from build123d import *

# Parameters (mm, degrees)
SKETCH1_R           = 3.1
BOSS_EXTRUDE1_DEPTH = 6


with BuildPart() as part:
    # Sketch1 → Boss-Extrude1 (new body)
    with BuildSketch(Plane(origin=(0, 0, 0), x_dir=(1, 0, 0), z_dir=(0, 1, 0))):
        with BuildLine():
            ThreePointArc((-31.599916308, 0.035666759), (-29.38660688, -5.361386604), (-24, -7.6))
            add(Edge.make_bspline(
                [(-24, -7.6), (-14.668264125, -7.61499575), (0.011178466, 17.82220608), (14.645907193, -7.566074292), (24, -7.6)],
                knots=[0, 0, 0, 0, 0.5, 1, 1, 1, 1], degree=3))
            ThreePointArc((24, -7.6), (29.374011537, -5.374011537), (31.6, 0))
            add(Edge.make_bspline(
                [(-31.599916308, 0.035666759), (-31.577855131, 6.453958953), (-15.873953038, 23.775800665), (16.019610489, 23.704017602), (31.552058953, 7.12035463), (31.6, 0)],
                knots=[0, 0, 0, 0, 0.447467305, 0.547467305, 1, 1, 1, 1], degree=3))
        make_face()
        with Locations(Location((-24, 0, 0), (0, 0, 270))):
            Circle(SKETCH1_R, mode=Mode.SUBTRACT)
        with Locations(Location((24, 0, 0), (0, 0, 270))):
            Circle(SKETCH1_R, mode=Mode.SUBTRACT)
        with Locations(Location((0, 16, 0), (0, 0, 270))):
            Circle(SKETCH1_R, mode=Mode.SUBTRACT)
    extrude(amount=BOSS_EXTRUDE1_DEPTH)


solid = part.part
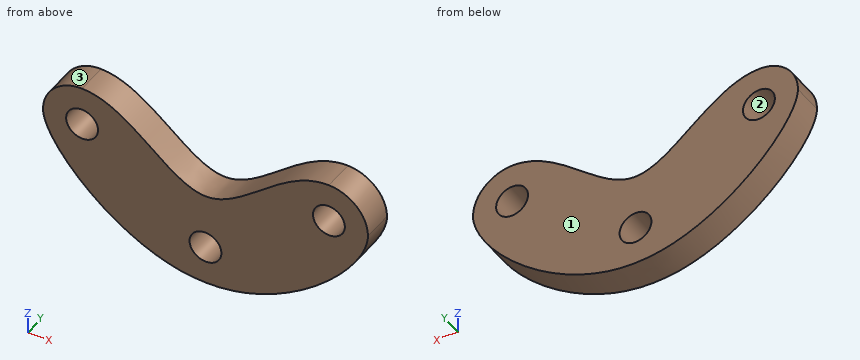
Read the model definition and answer for the solid it produces. Units are mm, in the model's axes. Face numbers are marked on the shaded views. Round coordinates to 2 decimals unless told otherwise and drop trailing zeros. Use a Markdown table: item, result.
(1) The part is cut by section A-A (y = 1.5). State how many separate pieces and enclosed holes the cut face has, then the cut area to 3 significant figures.
Reported:
| item | result |
|---|---|
| separate pieces | 1 |
| enclosed holes | 3 |
| area | 1,150 mm2 |
(2) Each of these flat-tipped pins is pushed along its axis until it touches: pin 1 Ø4 at (x, z) = (17, -13) entering from -Y; pin 2 Ø3.5 at (x, z) = (24, 0) entering from +Y; pin 3 Ø3 at (y, z) = (3.5, -10.5) entering from +X; pin 4 Ø1.5 at (y, z) = (1.5, -14) entering from +X. Where does it stop, or does it pass through?
Reported:
| item | result |
|---|---|
| pin 1 | y = 0 |
| pin 2 | through |
| pin 3 | x = 27.45 |
| pin 4 | x = 23.52 |
(3) The mould has two halves that part along X. Classify the marked faces 1, 2 and 3: released by +X, released by -X, zero draft, split by the parting line, or undercut.
Reported:
| item | result |
|---|---|
| face 1 | zero draft |
| face 2 | undercut |
| face 3 | released by -X |
(4) Straight lines are drawn through the part: line 1 along X through (y, z) = (1.9, -16); line 2 along Z through (x, y) = (22, 5.25); line 3 along X through (y, z) = (5.5, -14). For each, find the intervals that lie inside material, in ascending order. Write a range as [from, to].
Reported:
| item | result |
|---|---|
| line 1 | [-19.94, -3.1], [3.1, 20.26] |
| line 2 | [-14.6, -2.37], [2.37, 7.4] |
| line 3 | [-22.37, -2.37], [2.37, 22.7] |
